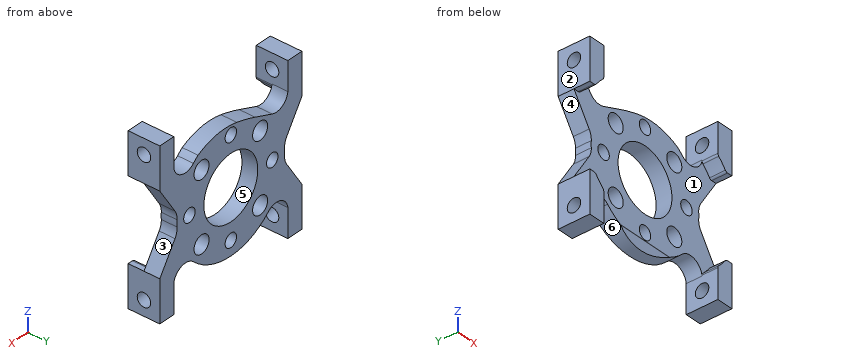
from build123d import *

# Parameters (mm, degrees)
SKETCH1_W                  = 33.528
SKETCH1_H                  = 33.02
BOSS_EXTRUDE1_DEPTH        = 3.175
CUT_EXTRUDE1_DEPTH         = 4.175
SKETCH3_W                  = 3.29438
SKETCH3_H                  = 8.37692
BOSS_EXTRUDE2_DEPTH        = 3.175
CUT_EXTRUDE2_DEPTH         = 7.35
SKETCH5_W                  = 3.29438
SKETCH5_H                  = 8.37692
BOSS_EXTRUDE3_DEPTH        = 3.175
CUT_EXTRUDE3_DEPTH         = 7.35
SKETCH7_W                  = 3.29438
SKETCH7_H                  = 8.37692
BOSS_EXTRUDE4_DEPTH        = 3.175
CUT_EXTRUDE4_DEPTH         = 7.35
SKETCH9_W                  = 3.29438
SKETCH9_H                  = 8.37692
BOSS_EXTRUDE5_DEPTH        = 3.175
CUT_EXTRUDE5_DEPTH         = 3.175
CUT_EXTRUDE6_DEPTH         = 3.175
CUT_EXTRUDE7_DEPTH         = 3.175
CUT_EXTRUDE8_DEPTH         = 3.175
HOLE1_D                    = 12.7254
HOLE1_DEPTH                = 3.175025
M2_5_CLEARANCE_HOLE1_D     = 2.7051
M2_5_CLEARANCE_HOLE1_DEPTH = 3.175025
M3_CLEARANCE_HOLE1_D       = 3.556
M3_CLEARANCE_HOLE1_DEPTH   = 3.175025
M2_5_CLEARANCE_HOLE2_D     = 2.7051
M2_5_CLEARANCE_HOLE2_DEPTH = 3.29438
M2_5_CLEARANCE_HOLE3_D     = 2.7051
M2_5_CLEARANCE_HOLE3_DEPTH = 3.29438
M2_5_CLEARANCE_HOLE4_D     = 2.7051
M2_5_CLEARANCE_HOLE4_DEPTH = 3.29443
FILLET1_R                  = 0.635
FILLET2_R                  = 3.175
CUT_EXTRUDE9_REACH         = 5.175
CUT_EXTRUDE12_REACH        = 7.42
SKETCH30_W                 = 14.449204344
SKETCH30_H                 = 9.791237154


with BuildPart() as part:
    # Sketch1 → Boss-Extrude1 (new body)
    with BuildSketch(Plane.XZ):
        Rectangle(SKETCH1_W, SKETCH1_H)
    extrude(amount=-BOSS_EXTRUDE1_DEPTH)

    # Sketch2 → Cut-Extrude1 (cut, through all)
    with BuildSketch(Plane(origin=(0, 3.175, 0), x_dir=(-1, 0, 0), z_dir=(0, 1, 0))):
        with BuildLine():
            Line((-13.46962, 16.51), (-13.46962, 10.753335779))
            ThreePointArc((-13.46962, 10.753335779), (-11.652039651, 8.508623021), (-8.8307675, 9.127296717))
            ThreePointArc((-8.8307675, 9.127296717), (0, 12.7), (8.8307675, 9.127296717))
            ThreePointArc((8.8307675, 9.127296717), (11.652039651, 8.508623021), (13.46962, 10.753335779))
            Line((13.46962, 10.753335779), (13.46962, 16.51))
            Line((13.46962, 16.51), (-13.46962, 16.51))
        make_face()
    extrude(amount=-CUT_EXTRUDE1_DEPTH, mode=Mode.SUBTRACT)

    # Sketch3 → Boss-Extrude2 (add)
    with BuildSketch(Plane.XZ):
        with Locations((-15.11681, 12.32154)):
            Rectangle(SKETCH3_W, SKETCH3_H)
    extrude(amount=BOSS_EXTRUDE2_DEPTH)

    # Sketch4 → Cut-Extrude2 (cut, through all)
    with BuildSketch(Plane(origin=(0, 3.175, 0), x_dir=(-1, 0, 0), z_dir=(0, 1, 0))):
        with BuildLine():
            Line((-16.764, 8.13308), (-16.764, -8.13308))
            Line((-16.764, -8.13308), (-12.593680427, -1.639882101))
            ThreePointArc((-12.593680427, -1.639882101), (-12.7, 0), (-12.593680427, 1.639882101))
            Line((-12.593680427, 1.639882101), (-16.764, 8.13308))
        make_face()
    extrude(amount=-CUT_EXTRUDE2_DEPTH, mode=Mode.SUBTRACT)

    # Sketch5 → Boss-Extrude3 (add)
    with BuildSketch(Plane.XZ):
        with Locations((15.11681, 12.32154)):
            Rectangle(SKETCH5_W, SKETCH5_H)
    extrude(amount=BOSS_EXTRUDE3_DEPTH)

    # Sketch6 → Cut-Extrude3 (cut, through all)
    with BuildSketch(Plane(origin=(0, 3.175, 0), x_dir=(-1, 0, 0), z_dir=(0, 1, 0))):
        with BuildLine():
            Line((13.46962, -16.51), (13.46962, -10.753335779))
            ThreePointArc((13.46962, -10.753335779), (11.652039651, -8.508623021), (8.8307675, -9.127296717))
            ThreePointArc((8.8307675, -9.127296717), (0, -12.7), (-8.8307675, -9.127296717))
            ThreePointArc((-8.8307675, -9.127296717), (-11.652039651, -8.508623021), (-13.46962, -10.753335779))
            Line((-13.46962, -10.753335779), (-13.46962, -16.51))
            Line((-13.46962, -16.51), (13.46962, -16.51))
        make_face()
    extrude(amount=-CUT_EXTRUDE3_DEPTH, mode=Mode.SUBTRACT)

    # Sketch7 → Boss-Extrude4 (add)
    with BuildSketch(Plane.XZ):
        with Locations((15.11681, -12.32154)):
            Rectangle(SKETCH7_W, SKETCH7_H)
    extrude(amount=BOSS_EXTRUDE4_DEPTH)

    # Sketch8 → Cut-Extrude4 (cut, through all)
    with BuildSketch(Plane(origin=(0, 3.175, 0), x_dir=(-1, 0, 0), z_dir=(0, 1, 0))):
        with BuildLine():
            Line((16.764, -8.13308), (16.764, 8.13308))
            Line((16.764, 8.13308), (12.593680427, 1.639882101))
            ThreePointArc((12.593680427, 1.639882101), (12.7, 0), (12.593680427, -1.639882101))
            Line((12.593680427, -1.639882101), (16.764, -8.13308))
        make_face()
    extrude(amount=-CUT_EXTRUDE4_DEPTH, mode=Mode.SUBTRACT)

    # Sketch9 → Boss-Extrude5 (add)
    with BuildSketch(Plane.XZ):
        with Locations((-15.11681, -12.32154)):
            Rectangle(SKETCH9_W, SKETCH9_H)
    extrude(amount=BOSS_EXTRUDE5_DEPTH)

    # Sketch10 → Cut-Extrude5 (cut)
    with BuildSketch(Plane.XZ.offset(3.175)):
        with BuildLine():
            Line((15.422429016, -8.13308), (13.46962, -8.13308))
            Line((13.46962, -8.13308), (13.46962, -10.329337463))
            ThreePointArc((13.46962, -10.329337463), (14.503938678, -9.282703292), (15.422429016, -8.13308))
        make_face()
    extrude(amount=-CUT_EXTRUDE5_DEPTH, mode=Mode.SUBTRACT)

    # Sketch11 → Cut-Extrude6 (cut)
    with BuildSketch(Plane.XZ.offset(3.175)):
        with BuildLine():
            Line((13.46962, 10.329337463), (13.46962, 8.13308))
            Line((13.46962, 8.13308), (15.422429016, 8.13308))
            ThreePointArc((15.422429016, 8.13308), (14.503938678, 9.282703292), (13.46962, 10.329337463))
        make_face()
    extrude(amount=-CUT_EXTRUDE6_DEPTH, mode=Mode.SUBTRACT)

    # Sketch12 → Cut-Extrude7 (cut)
    with BuildSketch(Plane.XZ.offset(3.175)):
        with BuildLine():
            Line((-15.422429016, 8.13308), (-13.46962, 8.13308))
            Line((-13.46962, 8.13308), (-13.46962, 10.329337463))
            ThreePointArc((-13.46962, 10.329337463), (-14.503938678, 9.282703292), (-15.422429016, 8.13308))
        make_face()
    extrude(amount=-CUT_EXTRUDE7_DEPTH, mode=Mode.SUBTRACT)

    # Sketch13 → Cut-Extrude8 (cut)
    with BuildSketch(Plane.XZ.offset(3.175)):
        with BuildLine():
            Line((-13.46962, -10.329337463), (-13.46962, -8.13308))
            Line((-13.46962, -8.13308), (-15.422429016, -8.13308))
            ThreePointArc((-15.422429016, -8.13308), (-14.503938678, -9.282703292), (-13.46962, -10.329337463))
        make_face()
    extrude(amount=-CUT_EXTRUDE8_DEPTH, mode=Mode.SUBTRACT)

    # Hole1
    with Locations(Plane(origin=(0, 0, 0), x_dir=(-1, 0, 0), z_dir=(0, -1, 0))):
        with Locations((0, 0)):
            Hole(HOLE1_D / 2, depth=HOLE1_DEPTH)

    # M2.5 Clearance Hole1
    with Locations(Plane(origin=(0, 0, 0), x_dir=(-1, 0, 0), z_dir=(0, -1, 0))):
        with Locations((0, -9.779), (9.779, 0), (0, 9.779), (-9.779, 0)):
            Hole(M2_5_CLEARANCE_HOLE1_D / 2, depth=M2_5_CLEARANCE_HOLE1_DEPTH)

    # M3 Clearance Hole1
    with Locations(Plane(origin=(0, 0, 0), x_dir=(-1, 0, 0), z_dir=(0, -1, 0))):
        with Locations((6.914797213, -6.914797213), (6.914797213, 6.914797213), (-6.914797213, 6.914797213), (-6.914797213, -6.914797213)):
            Hole(M3_CLEARANCE_HOLE1_D / 2, depth=M3_CLEARANCE_HOLE1_DEPTH)

    # M2.5 Clearance Hole2
    with Locations(Plane(origin=(16.764, 0, 0), x_dir=(0, 0, -1), z_dir=(1, 0, 0))):
        with Locations((13.470384182, 0)):
            Hole(M2_5_CLEARANCE_HOLE2_D / 2, depth=M2_5_CLEARANCE_HOLE2_DEPTH)

    # M2.5 Clearance Hole3
    with Locations(Plane.ZY.offset(-13.46962)):
        with Locations((13.470384182, 0)):
            Hole(M2_5_CLEARANCE_HOLE3_D / 2, depth=M2_5_CLEARANCE_HOLE3_DEPTH)

    # M2.5 Clearance Hole4
    with Locations(Plane(origin=(-13.46962, 0, 0), x_dir=(0, 0, -1), z_dir=(1, 0, 0))):
        with Locations((-13.470384182, 0), (13.470384182, 0)):
            Hole(M2_5_CLEARANCE_HOLE4_D / 2, depth=M2_5_CLEARANCE_HOLE4_DEPTH)

    # Fillet1
    fillet1_edges = [part.edges().sort_by_distance(p)[0] for p in [
        (-13.46962, -1.5875, -10.329337463),
        (-15.422429016, -1.5875, 8.13308),
        (15.422429016, -1.5875, -8.13308),
        (15.422429016, -1.5875, 8.13308),
        (13.46962, -1.5875, -10.329337463),
        (-13.46962, -1.5875, 10.329337463),
        (-15.422429016, -1.5875, -8.13308),
        (13.46962, -1.5875, 10.329337463),
    ]]
    fillet(fillet1_edges, radius=FILLET1_R)

    # Fillet2
    fillet2_edges = [part.edges().sort_by_distance(p)[0] for p in [
        (-12.593680427, 1.5875, -1.639882101),
        (12.593680427, 1.5875, -1.639882101),
        (-12.593680427, 1.5875, 1.639882101),
        (12.593680427, 1.5875, 1.639882101),
    ]]
    fillet(fillet2_edges, radius=FILLET2_R)

    # Sketch26 → Cut-Extrude9 (cut, up to next)
    with BuildSketch(Plane.XZ, mode=Mode.PRIVATE) as cut_extrude9_sk1:
        with BuildLine():
            Line((-9.767427274, 8.532567661), (-5.711894532, 10.070912798))
            ThreePointArc((-5.711894532, 10.070912798), (-3.581292847, 10.796642581), (-1.406006336, 11.374808519))
            ThreePointArc((-1.406006336, 11.374808519), (3.286728936, 11.571725124), (7.737358426, 10.070912798))
            ThreePointArc((7.737358426, 10.070912798), (-0.72214173, 12.679452327), (-8.8307675, 9.127296717))
            ThreePointArc((-8.8307675, 9.127296717), (-9.268785679, 8.78219321), (-9.767427274, 8.532567661))
        make_face()
    cut_extrude9_tool1 = extrude(cut_extrude9_sk1.sketch, amount=-CUT_EXTRUDE9_REACH, mode=Mode.PRIVATE) & part.part
    add(cut_extrude9_tool1.solids().sort_by_distance((-1.945542, 0, 11.38762))[0], mode=Mode.SUBTRACT)

    # Sketch30 → Cut-Extrude12 (cut, up to next)
    with BuildSketch(Plane(origin=(0, -5.02784088, -3.068243182), x_dir=(-1, 0, 0), z_dir=(0, -0.853608475, -0.520915129)), mode=Mode.PRIVATE) as cut_extrude12_sk1:
        with Locations((0.285206665, 14.086824926)):
            Rectangle(SKETCH30_W, SKETCH30_H)
    cut_extrude12_tool1 = extrude(cut_extrude12_sk1.sketch, amount=CUT_EXTRUDE12_REACH, mode=Mode.PRIVATE) & part.part
    add(cut_extrude12_tool1.solids().sort_by_distance((-0.285207, 2.310199, -15.092876))[0], mode=Mode.SUBTRACT)


solid = part.part
Here's how the part is built. I have some questions about the finished solid (model axes, mm). Face numbers are marked on the shaded views. A direction names the side the tool comes from. Give positions to 0.01 mm unless a question says otherwise; leave off trailing zeros. Loops run counter-clockwise (first coordinate to the right, second up) from the corner with the lowest first, then second, coordinate; pieces in that order, holes last. Notation, with made-up numbers: (62.25, 12) -> (102.25, 12) arc R7 cw to (102.25, 20) -> close; hole circle Ø10 at (-27, 79). An arc over 180 degrees is marked (long way). Answer as a JSON object with one key per item and string values. Group by question number.
Item 1: Imagine slicing it at B-B on x = 3. Write out the boundary of the cut face in (y, z) (3 decimals).
Item 2: Imagine slicing it at C-C on y = 2.75. Give the number of separate pieces and of enclosed holes in the cut face, then the cut area to 3 significant figures.
Item 3: Will these pins go through, and if not, where does the flat tip stop? pin 1 (1.5 mm diameter, centred on x = 3.5, y = -0.5, fed in from +Z); pin 2 (3.5 mm diameter, centred on x = 0, z = -9.779, fed in from -Y); pin 3 (3.5 mm diameter, centred on x = 9.779, z = 0, fed in from +Y) (3 decimals).
Item 4: Imagine slicing it at A-A on z = 0. Write out the boundary of the cut face in (x, y) (3 decimals), then the cut area to 3 significant figures.
Item 5: Imagine slicing it at D-D on x = 12. Write out the boundary of the cut face in (y, z) (3 decimals).
Item 6: Thinking about a two-plate mould opening in X: for the marked faces 3, 4, 5 and 6, which applies, pulls with the +X half, pulls with the -X half, needs draft (parallel to the pull), parting line crosses it, or undercut?
Item 7: On a 3-axis mill with a long thin cutter (end or side, diameter ignored), from which of +Z, -Z, +X, -X, +Y, -Y can I reach the whole of each face in a straight line? I mean the marked faces 1 and 2. Say none if no direction works.
Item 8: I need wall thicknesses on L1, parallel to X at y = 2.25, z = -6.5; L2, parallel to Z at x = 0, y = 1; L3, parallel to X at y = -2.5, z = 13. Which ranges of each line are inside material? Lowest first, please.
Answer list:
{
 "1": {"outline": "(0, -11.307) -> (0.631, -12.341) -> (3.175, -12.341) -> (3.175, -5.611) -> (0, -5.611) -> close; (0, 5.611) -> (3.175, 5.611) -> (3.175, 11.609) -> (0, 11.609) -> close"},
 "2": {"separate pieces": "1", "enclosed holes": "9", "area": "505 mm2"},
 "3": {"pin 1": "stops at z = 11.62", "pin 2": "stops at y = 0", "pin 3": "stops at y = 3.175"},
 "4": {"outline": "(-12.7, 0) -> (-11.132, 0) -> (-11.132, 3.175) -> (-12.7, 3.175) -> close; (-8.426, 0) -> (-6.363, 0) -> (-6.363, 3.175) -> (-8.426, 3.175) -> close; (6.363, 0) -> (8.426, 0) -> (8.426, 3.175) -> (6.363, 3.175) -> close; (11.132, 0) -> (12.7, 0) -> (12.7, 3.175) -> (11.132, 3.175) -> close", "area": "23.1 mm2"},
 "5": {"outline": "(0, -8.658) -> (3.175, -8.658) -> (3.175, 8.658) -> (0, 8.658) -> close"},
 "6": {"face 3": "pulls with the +X half", "face 4": "pulls with the -X half", "face 5": "undercut", "face 6": "undercut"},
 "7": {"face 1": "-Y", "face 2": "+Z, -Z, -X, +Y, -Y"},
 "8": {"L1": "x = -15.72 to -8.64, -5.19 to 5.19, 8.64 to 15.72", "L2": "z = -12.7 to -11.13, -8.43 to -6.36, 6.36 to 8.43, 11.13 to 11.62", "L3": "x = -16.76 to -13.47, 13.47 to 16.76"}
}
